The model under review builds one solid part; all positions refer to its coordinate system, in mm. Face numbers are marked on the shaded views. A direction names the side the tool comes from. Coordinates: 2 decimals unless noted, no trailing zeros. Order: outer loops, then holes, each group sorted by start corner. A loop starts at its lowest first (then second) coordinate and runs counter-clockwise, first axis right, second up.
```python
from build123d import *

# Parameters (mm, degrees)
SKETCH1_W           = 33.7
SKETCH1_H           = 6.3
SKETCH1_R           = 1.65
BOSS_EXTRUDE1_DEPTH = 2
SKETCH2_W           = 16
SKETCH2_H           = 3
BOSS_EXTRUDE2_DEPTH = 6
SKETCH3_R           = 1.65
CUT_EXTRUDE1_DEPTH  = 6
SKETCH4_W           = 16
SKETCH4_H           = 6
SKETCH4_R           = 1.65
BOSS_EXTRUDE3_DEPTH = 10


with BuildPart() as part:
    # Sketch1 → Boss-Extrude1 (new body)
    with BuildSketch(Plane.XY):
        with Locations((16.85, 3.15)):
            Rectangle(SKETCH1_W, SKETCH1_H)
        with Locations((3, 3.15)):
            Circle(SKETCH1_R, mode=Mode.SUBTRACT)
        with Locations((30.7, 3.15)):
            Circle(SKETCH1_R, mode=Mode.SUBTRACT)
    extrude(amount=BOSS_EXTRUDE1_DEPTH)

    # Sketch2 → Boss-Extrude2 (add)
    with BuildSketch(Plane.XY.offset(2)):
        with Locations((16.85, 1.5)):
            Rectangle(SKETCH2_W, SKETCH2_H)
    extrude(amount=BOSS_EXTRUDE2_DEPTH)

    # Sketch3 → Cut-Extrude1 (cut)
    with BuildSketch(Plane(origin=(0, 3, 0), x_dir=(1, 0, 0), z_dir=(0, 1, 0))):
        with Locations((12.85, -5)):
            Circle(SKETCH3_R)
        with Locations((20.85, -5)):
            Circle(SKETCH3_R)
    extrude(amount=-CUT_EXTRUDE1_DEPTH, mode=Mode.SUBTRACT)

    # Sketch4 → Boss-Extrude3 (add)
    with BuildSketch(Plane.XZ):
        with Locations((16.85, 5)):
            Rectangle(SKETCH4_W, SKETCH4_H)
        with Locations((12.85, 5)):
            Circle(SKETCH4_R, mode=Mode.SUBTRACT)
        with Locations((20.85, 5)):
            Circle(SKETCH4_R, mode=Mode.SUBTRACT)
    extrude(amount=BOSS_EXTRUDE3_DEPTH)


solid = part.part
```
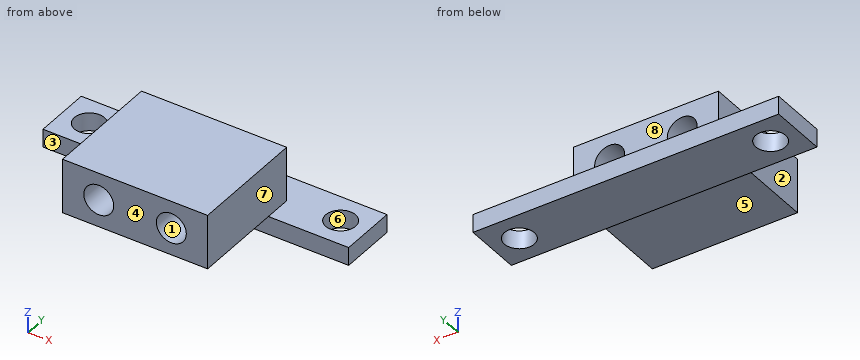
(1) For pin 1 Ø4 at (x, y) = (23, -7.5) entering from -Z; pin 2 Ø1.5 at (x, z) = (21, 4) entering from +Y; pin 3 Ø1 at (x, z) = (15.5, 1) entering from -Y, all flat-tipped, find the tip position at first contact; note any pin that passes through.
A:
pin 1: stops at z = 2
pin 2: stops at y = 3
pin 3: stops at y = 0
(2) We need section C-C, the plane y = -5.5. Write out the cut boundary in (x, z).
A:
outline: (8.85, 2) - (24.85, 2) - (24.85, 8) - (8.85, 8) - close; hole circle Ø3.3 at (12.85, 5); hole circle Ø3.3 at (20.85, 5)
(3) We need section A-A, the plane x = 12.85. Write out the cut boundary in (y, z), and give its area (3 significant figures).
A:
outline: (-10, 2) - (0, 2) - (0, 0) - (6.3, 0) - (6.3, 2) - (3, 2) - (3, 3.35) - (-10, 3.35) - close; (-10, 6.65) - (3, 6.65) - (3, 8) - (-10, 8) - close
area: 47.7 mm2
(4) Wall thickness on probe 1 along X at (y, z) = (-3.25, 5); probe 2 along X at (y, z) = (-7.75, 6.25); probe 3 along Y at (x, z) = (3, 1.5): over which ranges is each line inside the solid? List them lowest first.
A:
probe 1: x = 8.85 to 11.2, 14.5 to 19.2, 22.5 to 24.85
probe 2: x = 8.85 to 11.77, 13.93 to 19.77, 21.93 to 24.85
probe 3: y = 0 to 1.5, 4.8 to 6.3
(5) Draft analysis for pull direction X (two halves, no side actions). For the marked faces 1, 2 and 3, state which applies: released by +X, released by -X, zero draft, split by the parting line, or undercut.
A:
face 1: undercut
face 2: released by -X
face 3: zero draft
(6) We need section D-D, the plane x = 3. Write out the cut boundary in (y, z).
A:
outline: (0, 0) - (1.5, 0) - (1.5, 2) - (0, 2) - close; (4.8, 0) - (6.3, 0) - (6.3, 2) - (4.8, 2) - close
(7) Machinability: for the marked faces 4, 5, 6, 7 and 8, which of the approach directions +Z, -Z, +X, -X, +Y, -Y give a long, thin tool a straight path to every point of the face, cutting with its end or side? Answer none if there is none.
A:
face 4: +Z, -Z, +X, -X, -Y
face 5: -Z, +X, -X, -Y
face 6: +Z, -Z
face 7: +Z, +X, +Y, -Y
face 8: +Z, +X, -X, +Y
(8) We need section B-B, the plane z = 1.5. Write out the cut boundary in (x, y), and give its area (3 significant figures).
A:
outline: (0, 0) - (33.7, 0) - (33.7, 6.3) - (0, 6.3) - close; hole circle Ø3.3 at (3, 3.15); hole circle Ø3.3 at (30.7, 3.15)
area: 195 mm2
